Input: part model. Units: mm. Frame: model coordinates. Face numbers are marked on the shaded views. Coordinates: 2 decimals unless noted, no trailing zeros. Order: outer loops, then holes, each group sorted by start corner. A loop starts at its lowest first (then second) coordinate and runs counter-clockwise, first axis right, second up. Notation, with made-up numbers: (-37.75, 69.5) - (-4.75, 69.5) arc R21 ccw to (-4.75, 100.5) - close; hole circle Ø1 at (46, 67.5). An arc over 180 degrees is marked (long way). One line per question, with ' | ' between items.
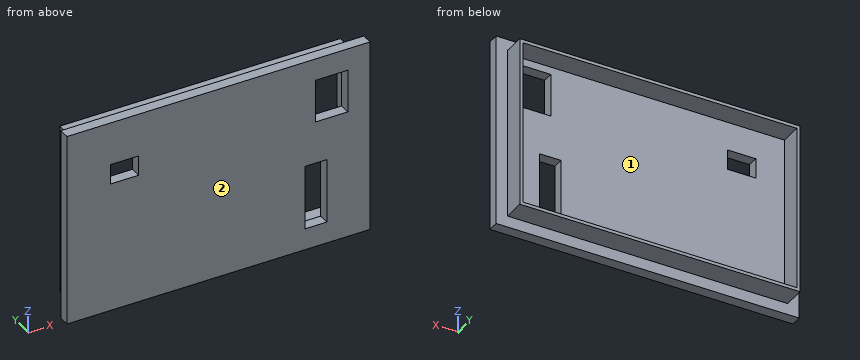
from build123d import *

# Parameters (mm, degrees)
CROQUIS1_W              = 140
CROQUIS1_H              = 90
SALIENTE_EXTRUIR1_DEPTH = 5
CROQUIS2_W              = 129.5
CROQUIS2_H              = 79.5
CROQUIS2_W_2            = 126.5
CROQUIS2_H_2            = 76.5
SALIENTE_EXTRUIR2_DEPTH = 10
CROQUIS3_W              = 15
CROQUIS3_H              = 20
CORTAR_EXTRUIR1_DEPTH   = 84.815273071
CROQUIS4_W              = 13.1
CROQUIS4_H              = 9.3
CORTAR_EXTRUIR2_DEPTH   = 85.557672626
CROQUIS5_W              = 10
CROQUIS5_H              = 30
CORTAR_EXTRUIR3_DEPTH   = 85.557672626


with BuildPart() as part:
    # Croquis1 → Saliente-Extruir1 (new body)
    with BuildSketch(Plane(origin=(0, 0, 0), x_dir=(1, 0, 0), z_dir=(0, 1, 0))):
        Rectangle(CROQUIS1_W, CROQUIS1_H)
    extrude(amount=SALIENTE_EXTRUIR1_DEPTH)

    # Croquis2 → Saliente-Extruir2 (add)
    with BuildSketch(Plane(origin=(0, 5, 0), x_dir=(1, 0, 0), z_dir=(0, 1, 0))):
        Rectangle(CROQUIS2_W, CROQUIS2_H)
        Rectangle(CROQUIS2_W_2, CROQUIS2_H_2, mode=Mode.SUBTRACT)
    extrude(amount=SALIENTE_EXTRUIR2_DEPTH)

    # Croquis3 → Cortar-Extruir1 (cut, through all)
    with BuildSketch(Plane(origin=(0, 5, 0), x_dir=(1, 0, 0), z_dir=(0, 1, 0))):
        with Locations((52.25, -24.75)):
            Rectangle(CROQUIS3_W, CROQUIS3_H)
    extrude(amount=-CORTAR_EXTRUIR1_DEPTH, mode=Mode.SUBTRACT)

    # Croquis4 → Cortar-Extruir2 (cut, through all)
    with BuildSketch(Plane.XZ):
        with Locations((-43.45, 20.35)):
            Rectangle(CROQUIS4_W, CROQUIS4_H)
    extrude(amount=-CORTAR_EXTRUIR2_DEPTH, mode=Mode.SUBTRACT)

    # Croquis5 → Cortar-Extruir3 (cut, through all)
    with BuildSketch(Plane.XZ):
        with Locations((45, -20)):
            Rectangle(CROQUIS5_W, CROQUIS5_H)
    extrude(amount=-CORTAR_EXTRUIR3_DEPTH, mode=Mode.SUBTRACT)


solid = part.part
Item 1: Section B-B on x = -40. Return the cut outline in (y, z).
Data:
outline: (0, -45) - (5, -45) - (5, -39.75) - (15, -39.75) - (15, -38.25) - (5, -38.25) - (5, 15.7) - (0, 15.7) - close; (0, 25) - (5, 25) - (5, 38.25) - (15, 38.25) - (15, 39.75) - (5, 39.75) - (5, 45) - (0, 45) - close
Item 2: Ray query, line 1 (X direction, y = 2, z = 17); line 2 (X direction, y = 13.5, z = 9); line 3 (Z direction, x = 44, y = 5.5). Return the intervals inside material, ascending.
Data:
line 1: -70 to -50, -36.9 to 44.75, 59.75 to 70 | line 2: -64.75 to -63.25, 63.25 to 64.75 | line 3: -39.75 to -38.25, 38.25 to 39.75
Item 3: Section C-C on y = 2. Return the cut outline in (x, z).
Data:
outline: (-70, -45) - (70, -45) - (70, 45) - (-70, 45) - close; hole (-50, 15.7) - (-36.9, 15.7) - (-36.9, 25) - (-50, 25) - close; hole (40, -35) - (50, -35) - (50, -5) - (40, -5) - close; hole (44.75, 14.75) - (59.75, 14.75) - (59.75, 34.75) - (44.75, 34.75) - close
Item 4: Section D-D on z = 21.5. Return the cut outline in (x, y).
Data:
outline: (-70, 0) - (-50, 0) - (-50, 5) - (-63.25, 5) - (-63.25, 15) - (-64.75, 15) - (-64.75, 5) - (-70, 5) - close; (-36.9, 0) - (44.75, 0) - (44.75, 5) - (-36.9, 5) - close; (59.75, 0) - (70, 0) - (70, 5) - (64.75, 5) - (64.75, 15) - (63.25, 15) - (63.25, 5) - (59.75, 5) - close
Item 5: Contact query for flat-ended pins moving along their axis: P1, Ø5, axis at y = 11, z = -16.5, coming from the -X side; P2, Ø1.5, axis at x = -13.5, y = 11.5, coming from the -Z side; P3, Ø12, axis at x = 45.5, z = 30.5, coming from the +Y side. Output: stop coordinate, or through.
Data:
P1: x = -64.75 | P2: z = -39.75 | P3: y = 5
Item 6: Section A-A on z = -6.5. Return the cut outline in (x, y), and give its area (3 significant figures).
Data:
outline: (-70, 0) - (40, 0) - (40, 5) - (-63.25, 5) - (-63.25, 15) - (-64.75, 15) - (-64.75, 5) - (-70, 5) - close; (50, 0) - (70, 0) - (70, 5) - (64.75, 5) - (64.75, 15) - (63.25, 15) - (63.25, 5) - (50, 5) - close | area: 680 mm^2
Item 7: Draft query along Z for the marked faces 1 and 2. Return one class per face: released by +Z, released by -Z, zero draft, split by the parting line, or undercut.
Data:
face 1: undercut | face 2: zero draft
